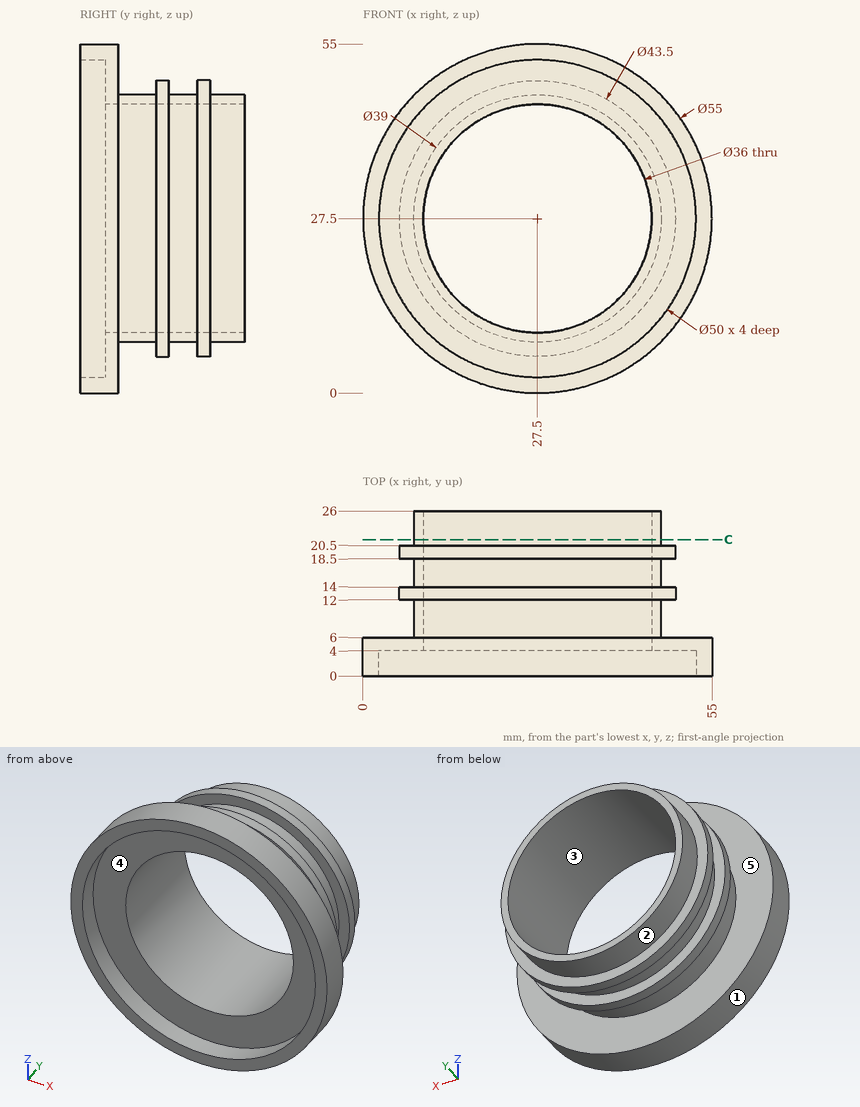
For this review, use the dimensioned drawing (mm, ordinates from the lowest corner) and the shaded views. A direction names the side the tool comes from. Give positions to 0.01 mm unless a question says otherwise; leave off trailing zeros. Order: outer loops, then holes, each group sorted by start corner. A loop starts at its lowest first (then second) coordinate and runs counter-clockwise, first axis right, second up. Notation, with made-up numbers: (77, -35.75) - (82, -35.75) arc R13 cw to (82, -20.75) - close; hole circle Ø9 at (48.5, 20). An arc over 180 degrees is marked (long way). Use a Markdown table: item, result. Add a question column.
(1) Machinability: for the marked faces 1 and 2, which of the approach directions +Z, -Z, +X, -X, +Y, -Y give a long, thin tool a straight path to every point of the face, cutting with its end or side? Answer none if there is none.
(2) Clearance check with flat-ended pins moving along their axes: P1, Ø13, axis at x = 18.5, z = 17.5, coming from the -Y side; P2, Ø12, axis at y = 13, z = 12, coming from the -X side; P3, Ø3, axis at y = 4.5, z = 34.5, coming from the -X side; P4, Ø13, axis at x = 18.5, z = 32, coming from the +Y side. State where each tip first meets the part, or that it passes through.
(3) Add section C-C on y = 21.5. Give the boundary of the cut face in (x, z), then the cut area to 3 significant figures.
(4) Mouldability with a two-part tool opening along Y and no side actions: class the marked faces 3, 4 and 5 as +Y half, -Y half, draft (parallel to the pull), parting line (faces both ways), or undercut.
(5) Wall thickness on probe 1 along Y at (x, z) = (43, 42); probe 2 along X at (y, z) = (9, 27.5); probe 3 along Z at (x, y) = (27, 24.5): over which ranges is each line inside the solid? List them lowest first. Write a range as [from, to].
Report:
| question | item | result |
|---|---|---|
| 1 | face 1 | +Y, -Y |
| 1 | face 2 | +Y |
| 2 | P1 | stops at y = 4 |
| 2 | P2 | stops at x = 7.93 |
| 2 | P3 | stops at x = 0.56 |
| 2 | P4 | passes through |
| 3 | outline | circle Ø39 at (27.5, 27.5); hole circle Ø36 at (27.5, 27.5) |
| 3 | area | 177 mm² |
| 4 | face 3 | draft |
| 4 | face 4 | -Y half |
| 4 | face 5 | undercut |
| 5 | probe 1 | y = [4, 6], [12, 14], [18.5, 20.5] |
| 5 | probe 2 | x = [8, 9.5], [45.5, 47] |
| 5 | probe 3 | z = [8.01, 9.51], [45.49, 46.99] |
